from build123d import *

# Parameters (mm, degrees)
SKETCH1_R           = 3.175
BOSS_EXTRUDE1_DEPTH = 12.7
BOSS_EXTRUDE8_DEPTH = 19.05
CUT_EXTRUDE3_DEPTH  = 41.148
BOSS_EXTRUDE9_DEPTH = 25.4


with BuildPart() as part:
    # Sketch1 → Boss-Extrude1 (new body)
    with BuildSketch(Plane.XY):
        with BuildLine():
            Line((299.870251741, -63.185614448), (503.070251741, -63.185614448))
            ThreePointArc((503.070251741, -63.185614448), (518.945251741, -79.060614448), (503.070251741, -94.935614448))
            Line((503.070251741, -94.935614448), (299.870251741, -94.935614448))
            ThreePointArc((299.870251741, -94.935614448), (283.995251741, -79.060614448), (299.870251741, -63.185614448))
        make_face()
        with Locations((299.870251741, -79.060614448)):
            Circle(SKETCH1_R, mode=Mode.SUBTRACT)
        with Locations((503.070251741, -79.060614448)):
            Circle(SKETCH1_R, mode=Mode.SUBTRACT)
    extrude(amount=BOSS_EXTRUDE1_DEPTH)

    # Sketch7 → Boss-Extrude8 (add)
    with BuildSketch(Plane.XY.offset(12.7)):
        with BuildLine():
            Line((310.030251741, -66.360614448), (312.570251741, -66.360614448))
            Line((312.570251741, -66.360614448), (322.730251741, -66.360614448))
            Line((322.730251741, -66.360614448), (322.730251741, -91.760614448))
            Line((322.730251741, -91.760614448), (310.030251741, -91.760614448))
            Line((310.030251741, -91.760614448), (289.710251741, -91.760614448))
            ThreePointArc((289.710251741, -91.760614448), (287.914200517, -91.016665672), (287.170251741, -89.220614448))
            Line((287.170251741, -89.220614448), (287.170251741, -68.900614448))
            ThreePointArc((287.170251741, -68.900614448), (287.914200517, -67.104563223), (289.710251741, -66.360614448))
            Line((289.710251741, -66.360614448), (310.030251741, -66.360614448))
        make_face()
    extrude(amount=BOSS_EXTRUDE8_DEPTH)

    # Sketch8 → Cut-Extrude3 (cut)
    with BuildSketch(Plane(origin=(0, -66.360614448, 0), x_dir=(1, 0, 0), z_dir=(0, 1, 0))):
        with BuildLine():
            Line((287.170251741, -12.7), (317.904251741, -12.7))
            ThreePointArc((317.904251741, -12.7), (317.648023156, -21.431345807), (311.300251741, -27.432))
            Line((311.300251741, -27.432), (287.170251741, -27.432))
            Line((287.170251741, -27.432), (287.170251741, -12.7))
        make_face()
    extrude(amount=-CUT_EXTRUDE3_DEPTH, mode=Mode.SUBTRACT)

    # Sketch9 → Boss-Extrude9 (add)
    with BuildSketch(Plane(origin=(0, -66.360614448, 0), x_dir=(1, 0, 0), z_dir=(0, 1, 0))):
        Polygon((322.730251741, -31.75), (349.936471269, -12.7), (322.730251741, -12.7), align=None)
    extrude(amount=-BOSS_EXTRUDE9_DEPTH)


solid = part.part
Part model, mm, in its own coordinate system. A direction names the side the tool comes from. Give positions to 0.01 mm unless a question says otherwise; leave off trailing zeros. Loops run counter-clockwise (first coordinate to the right, second up) from the corner with the lowest first, then second, coordinate; pieces in that order, holes last. Notation, with made-up numbers: (-13.75, -2.75) -> (26.25, -2.75) arc R31 cw to (26.25, 33.25) -> close; hole circle Ø11 at (41.25, 78.25). An arc over 180 degrees is marked (long way). Write each question's results on one line, items separated by ' | '. Start each with the question number.
Q1. Band-saw the part on C-C on y = -85. List the corners of the cut face in (x, z), plus the area to 3 significant figures.
Q2. Band-saw the part on D-D on z = 19.5. List the corners of the cut face in (x, y).
Q3. Pin check, flat tips, straight feed: P1, Ø5, axis at y = -86.5, z = 14, coming from the -X side; P2, Ø9.5, axis at x = 327, z = 19, coming from the +Y side; P3, Ø12, axis at y = -68.5, z = 23.5, coming from the -X side. Stop position of each tip, or through.
Q4. Pull direction X, two halves, no side cores. Call faces 1 (the face through (319, -66.361, 22)), 2 (the face through (287.17, -79, 30)), 3 (the face through (296.7, -78.9, 6.3)): +X half, -X half, draft (parallel to the pull), parting line (faces both ways), or undercut.
Q5. Which spindle directions (+Z, -Z, +X, -X, +Y, -Y) get a long thin tool onto all of the face, cutting with end or side? Do faces 4 (the face through (336.14, -78.88, 22.36)), 5 (the face through (299, -79, 27.432)), 6 (the face through (284, -79.4, 6.3)), 7 (the face through (319, -91.761, 22)). Say none if no direction does.
Q6. Wall check: L1, parallel to Z at x = 299, y = -73; L2, parallel to Z at x = 356.5, y = -67.5; L3, parallel to Y at x = 316.5, z = 26.5. Give the ranges that are in metal, low to high.
Q7. Band-saw the part on A-A on z = 10. List the corners of the cut face in (x, y) (3 decimals), plus the area to 3 significant figures.
Q8. Band-saw the part on B-B on x = 354.5. List the corners of the cut face in (y, z), plus the area to 3 significant figures.
Results are:
1) outline: (285.15, 0) -> (517.79, 0) -> (517.79, 12.7) -> (349.94, 12.7) -> (322.73, 31.75) -> (287.17, 31.75) -> (287.17, 27.43) -> (311.3, 27.43) arc R11.43 cw to (317.9, 12.7) -> (285.15, 12.7) -> close | area: 3,450 mm²
2) outline: (318.31, -91.76) -> (340.23, -91.76) -> (340.23, -66.36) -> (318.31, -66.36) -> close
3) P1: stops at x = 284.91 | P2: stops at y = -66.36 | P3: stops at x = 287.17
4) face 1: draft | face 2: -X half | face 3: undercut
5) face 4: +Z, +X, +Y, -Y | face 5: -X, +Y, -Y | face 6: -Z, -X | face 7: +Z, +X, -X, -Y
6) L1: z = 0 to 12.7, 27.43 to 31.75 | L2: z = 0 to 12.7 | L3: y = -91.76 to -66.36
7) outline: (299.87, -94.936) -> (503.07, -94.936) arc R15.875 ccw to (503.07, -63.186) -> (299.87, -63.186) arc R15.875 ccw to start; hole circle Ø6.35 at (299.87, -79.061); hole circle Ø6.35 at (503.07, -79.061) | area: 7,180 mm²
8) outline: (-94.94, 0) -> (-63.19, 0) -> (-63.19, 12.7) -> (-94.94, 12.7) -> close | area: 403 mm²
